from build123d import *

# Parameters (mm, degrees)
F1_DEPTH       = 152.4
F3_D           = 9.525
F3_CSINK_D     = 19.8628
F3_CSINK_ANGLE = 82
F4_R           = 4.7625
F5_DEPTH       = 1.27
F7_DEPTH       = 76.201


# Not quite as in the source:
# - a length typed as a fraction of an inch, garbled in the dataset ("3 / 203.2 mm" for 3/8 in), is restored
# - a feature names something its author has since deleted; it is built from what else it names


with BuildPart() as f1:
    # F0 (on Right) → F1 (new body)
    with BuildSketch(Plane.YZ):
        Polygon((76.2, -6.35), (76.2, 0), (0, 0), (0, -76.2), (6.35, -76.2), (6.35, -6.35), align=None)
    extrude(amount=F1_DEPTH)

    # F3 (through all)
    with Locations(Plane(origin=(0, 0, -6.35), x_dir=(1, 0, 0), z_dir=(0, 0, -1))):
        with Locations((76.2, -38.1)):
            CounterSinkHole(F3_D / 2, F3_CSINK_D / 2, counter_sink_angle=F3_CSINK_ANGLE)

    # F4 (on face) → F5 (cut)
    with BuildSketch(Plane.XY):
        with BuildLine():
            Line((111.125, 63.5), (41.275, 63.5))
            ThreePointArc((41.275, 63.5), (39.0299359697, 62.5700640303), (38.1, 60.325))
            Line((38.1, 60.325), (38.1, 15.875))
            ThreePointArc((38.1, 15.875), (39.0299359697, 13.6299359697), (41.275, 12.7))
            Line((41.275, 12.7), (111.125, 12.7))
            ThreePointArc((111.125, 12.7), (113.3700640303, 13.6299359697), (114.3, 15.875))
            Line((114.3, 15.875), (114.3, 60.325))
            ThreePointArc((114.3, 60.325), (113.3700640303, 62.5700640303), (111.125, 63.5))
        make_face()
        with Locations((76.2, 38.1)):
            Circle(F4_R, mode=Mode.SUBTRACT)
    extrude(amount=-F5_DEPTH, mode=Mode.SUBTRACT)

    # F6 (on face) → F7 (cut, through all)
    with BuildSketch(Plane.XZ):
        with BuildLine():
            Line((71.4375, -47.625), (71.4375, -53.975))
            ThreePointArc((71.4375, -53.975), (76.2, -58.7375), (80.9625, -53.975))
            Line((80.9625, -53.975), (80.9625, -47.625))
            ThreePointArc((80.9625, -47.625), (76.2, -42.8625), (71.4375, -47.625))
        make_face()
    extrude(amount=-F7_DEPTH, mode=Mode.SUBTRACT)


solid = f1.part
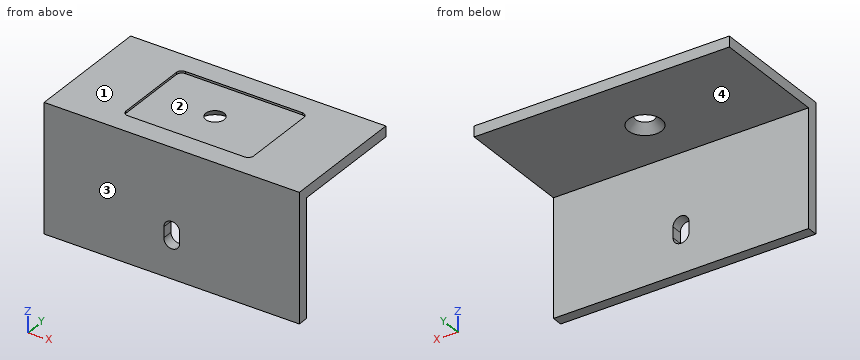
The listing builds one solid part. Answer for the finished solid, in the listing's coordinates (mm). Face numbers are marked on the shaded views. A direction names the side the tool comes from. Round coordinates to 2 decimals unless told otherwise and drop trailing zeros. Order: outer loops, then holes, each group sorted by start corner. A loop starts at its lowest first (then second) coordinate and runs counter-clockwise, first axis right, second up. Notation, with made-up numbers: (83, -38) - (90, -38) arc R9 cw to (90, -27) - close; hole circle Ø11 at (20, -6.75). An arc over 180 degrees is marked (long way). Write item = value, one per line. Start each with the question number.
1) Given pin 1 (15 mm diameter, centred on x = 71.5, y = 26.5, fed in from +Z); pin 2 (21 mm diameter, centred on x = 61.5, z = -24.5, fed in from +Y); pin 3 (1.5 mm diameter, centred on x = 85.5, y = 9.5, fed in from -Z), each flat-ended and moving along its own axis, determine where each tip first touches the part or whether it passes through.
2) For the marked faces 3 and 4, determine the directions among +Z, -Z, +X, -X, +Y, -Y from which every point of the face is accessible in a straight line to the end or side of a thin tool.
3) For a pull along X with two mould halves and no side action, classify the marked faces 1 and 2 as released by +X, released by -X, zero draft, split by the parting line, or undercut.
4) Section A-A, the plane x = 76.2 is taken. Write down the section's boundary in (y, z), plus the area to 3 significant figures.
5) Section C-C, the plane y = 38.1 is taken. Write down the section's boundary in (x, z).
6) Straight lines are drawn through the part: L1, parallel to Y at x = 44, z = -58.5; L2, parallel to Z at x = 49, y = 63; L3, parallel to Z at x = 17, y = 19.5. For each, find the intervals that lie inside material, in ascending order.
7) Section D-D, the plane y = 56 is taken. Write down the section's boundary in (x, z), plus the area to 3 significant figures.
8) Section B-B, the plane x = 52.5 is taken. Write down the section's boundary in (y, z), plus the area to 3 significant figures.
Results list:
q1.pin_1 = -1.27
q1.pin_2 = 6.35
q1.pin_3 = -6.35
q2.face_3 = +Z, -Z, +X, -X, -Y
q2.face_4 = -Z, +X, -X, +Y
q3.face_1 = zero draft
q3.face_2 = undercut
q4.outline = (0, -76.2) - (6.35, -76.2) - (6.35, -58.74) - (0, -58.74) - close; (0, -42.86) - (6.35, -42.86) - (6.35, -6.35) - (28.17, -6.35) - (32.58, -1.27) - (12.7, -1.27) - (12.7, 0) - (0, 0) - close; (43.62, -1.27) - (48.03, -6.35) - (76.2, -6.35) - (76.2, 0) - (63.5, 0) - (63.5, -1.27) - close
q4.area = 684 mm^2
q5.outline = (0, -6.35) - (66.27, -6.35) - (70.68, -1.27) - (38.1, -1.27) - (38.1, 0) - (0, 0) - close; (81.72, -1.27) - (86.13, -6.35) - (152.4, -6.35) - (152.4, 0) - (114.3, 0) - (114.3, -1.27) - close
q6.L1 = 0 to 6.35
q6.L2 = -6.35 to -1.27
q6.L3 = -6.35 to 0
q7.outline = (0, -6.35) - (152.4, -6.35) - (152.4, 0) - (114.3, 0) - (114.3, -1.27) - (38.1, -1.27) - (38.1, 0) - (0, 0) - close
q7.area = 871 mm^2
q8.outline = (0, -76.2) - (6.35, -76.2) - (6.35, -6.35) - (76.2, -6.35) - (76.2, 0) - (63.5, 0) - (63.5, -1.27) - (12.7, -1.27) - (12.7, 0) - (0, 0) - close
q8.area = 863 mm^2
